Check sheet for the modelled part. Datum: model origin and axes. Units: mm. Give positions to 0.01 mm unless a question says otherwise; leave off trailing zeros. Order: outer loops, then holes, each group sorted by start corner. A loop starts at its lowest first (then second) coordinate and runs counter-clockwise, first axis right, second up.
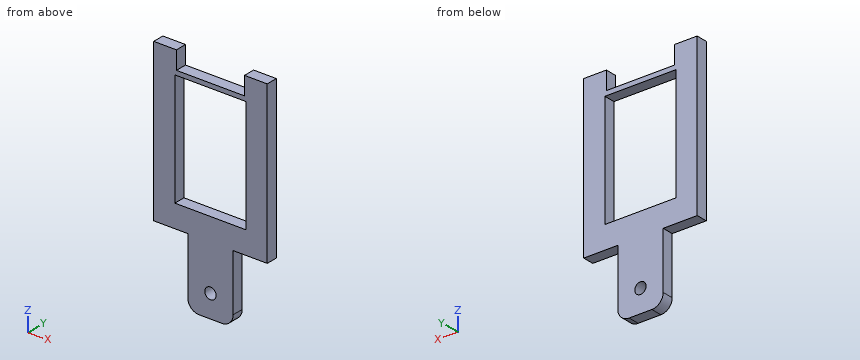
from build123d import *

# Parameters (mm, degrees)
SKETCH1_R           = 0.635
SKETCH1_W           = 7.96592112
SKETCH1_H           = 12.7
BOSS_EXTRUDE1_DEPTH = 1.27


with BuildPart() as part:
    # Sketch1 → Boss-Extrude1 (new body)
    with BuildSketch(Plane(origin=(0, 0, 0), x_dir=(1, 0, 0), z_dir=(0, 1, 0))):
        with BuildLine():
            Line((6.35, -8.89), (6.35, 8.89))
            Line((6.35, 8.89), (2.54, 8.89))
            Line((2.54, 8.89), (2.54, 15.24))
            ThreePointArc((2.54, 15.24), (2.168025612, 16.138025612), (1.27, 16.51))
            Line((1.27, 16.51), (-1.27, 16.51))
            ThreePointArc((-1.27, 16.51), (-2.168025612, 16.138025612), (-2.54, 15.24))
            Line((-2.54, 15.24), (-2.54, 8.89))
            Line((-2.54, 8.89), (-6.35, 8.89))
            Line((-6.35, 8.89), (-6.35, -8.89))
            Line((-6.35, -8.89), (-3.81, -8.89))
            Line((-3.81, -8.89), (-3.81, -6.858))
            Line((-3.81, -6.858), (3.81, -6.858))
            Line((3.81, -6.858), (3.81, -8.89))
            Line((3.81, -8.89), (6.35, -8.89))
        make_face()
        with Locations((0, 13.97)):
            Circle(SKETCH1_R, mode=Mode.SUBTRACT)
        Rectangle(SKETCH1_W, SKETCH1_H, mode=Mode.SUBTRACT)
    extrude(amount=BOSS_EXTRUDE1_DEPTH)


solid = part.part
1) Section check C-C, the plane x = 0. Record the cut outline in (y, z) (3 decimals), then the cut area to 3 significant figures.
Recorded:
outline: (0, -16.51) - (1.27, -16.51) - (1.27, -14.605) - (0, -14.605) - close; (0, -13.335) - (1.27, -13.335) - (1.27, -6.35) - (0, -6.35) - close; (0, 6.35) - (1.27, 6.35) - (1.27, 6.858) - (0, 6.858) - close
area: 11.9 mm2
2) Depth check by flat-ended pin: pin 1 Ø5 at (x, z) = (4.5, -10.5) entering from +Y; pin 2 Ø0.6 at (y, z) = (1, -13.5) entering from +X; pin 3 Ø0.6 at (x, y) = (1.5, 0.5) entering from +Z. Enter the tip coordinate at first touch or a pass-through.
Recorded:
pin 1: stops at y = 1.27
pin 2: stops at x = 2.54
pin 3: stops at z = 6.86
3) Material ranges on L1, parallel to Z at x = 0, y = 0.7 (3 decimals); L2, parallel to Z at x = 3.5, y = 0.95; L3, parallel to X at y = 1.2, z = 7, recorded low to high.
Recorded:
L1: z = -16.51 to -14.605, -13.335 to -6.35, 6.35 to 6.858
L2: z = -8.89 to -6.35, 6.35 to 6.86
L3: x = -6.35 to -3.81, 3.81 to 6.35
4) Section check D-D, the plane y = 0.65. Record the cut outline in (x, z) (3 decimals).
Recorded:
outline: (-6.35, -8.89) - (-2.54, -8.89) - (-2.54, -15.24) arc R1.27 ccw to (-1.27, -16.51) - (1.27, -16.51) arc R1.27 ccw to (2.54, -15.24) - (2.54, -8.89) - (6.35, -8.89) - (6.35, 8.89) - (3.81, 8.89) - (3.81, 6.858) - (-3.81, 6.858) - (-3.81, 8.89) - (-6.35, 8.89) - close; hole (-3.983, -6.35) - (3.983, -6.35) - (3.983, 6.35) - (-3.983, 6.35) - close; hole circle Ø1.27 at (0, -13.97)
5) Section check A-A, the plane x = -3. Record the cut outline in (y, z), then the cut area to 3 significant figures.
Recorded:
outline: (0, -8.89) - (1.27, -8.89) - (1.27, -6.35) - (0, -6.35) - close; (0, 6.35) - (1.27, 6.35) - (1.27, 6.86) - (0, 6.86) - close
area: 3.87 mm2
6) Section check B-B, the plane z = 4.75. Record the cut outline in (x, y), then the cut area to 3 significant figures.
Recorded:
outline: (-6.35, 0) - (-3.98, 0) - (-3.98, 1.27) - (-6.35, 1.27) - close; (3.98, 0) - (6.35, 0) - (6.35, 1.27) - (3.98, 1.27) - close
area: 6.01 mm2
